Check sheet for the drawn part. Datum: minimum x, y, z corner. Units: mm. Give positions to 0.01 mm unless a question says otherwise; leave off trailing zeros. Order: outer loops, then holes, each group sorted by start corner. A loop starts at its lowest first (then second) coordinate and runs counter-clockwise, first axis right, second up. Notation, with made-up numbers: (-0.75, -12.75) -> (8.25, -12.75) arc R30 ccw to (8.25, 13.25) -> close; hole circle Ø1 at (53.5, 21.5). An arc over 180 degrees is marked (long way). Answer in a Markdown table with one row per item. Add a question column.
(1) Cross-section at B-B (x = 71.5). Record the cut outline in (y, z), then the cut area to 3 significant figures.
(2) Cross-section at C-C (z = 36). Record the cut outline in (x, y), then the cut area to 3 significant figures.
(3) Release check for a two-part mould opening along X. For the marked faces 1 and 2 record: released by +X, released by -X, zero draft, split by the parting line, or undercut.
(4) Cross-section at D-D (z = 46.5). Record the cut outline in (x, y), then the cut area to 3 significant figures.
(5) Go/stop test with flat-tipped pins: pin 1 (2 mm diameter, centred on x = 32.5, y = 1.5, fed in from -Z); pin 2 (5.5 mm diameter, centred on x = 71.5, z = 46.5, fed in from +Y); pin 3 (2 mm diameter, centred on x = 26.5, z = 25.5, fed in from +Y). Record where each tip stops, or that it passes through.
(6) Thickness scan on L1, parallel to X at y = 3.6, z = 46.5; L2, parallel to X at y = 3, z = 38; L3, parallel to Z at x = 21.5, y = 5.5. Record the ranges inside material, lowest first. Write a range as [from, to].
(7) Cross-section at A-A (y = 3). State how many separate pieces and enclosed holes the cut face has, then the cut area to 3 significant figures.
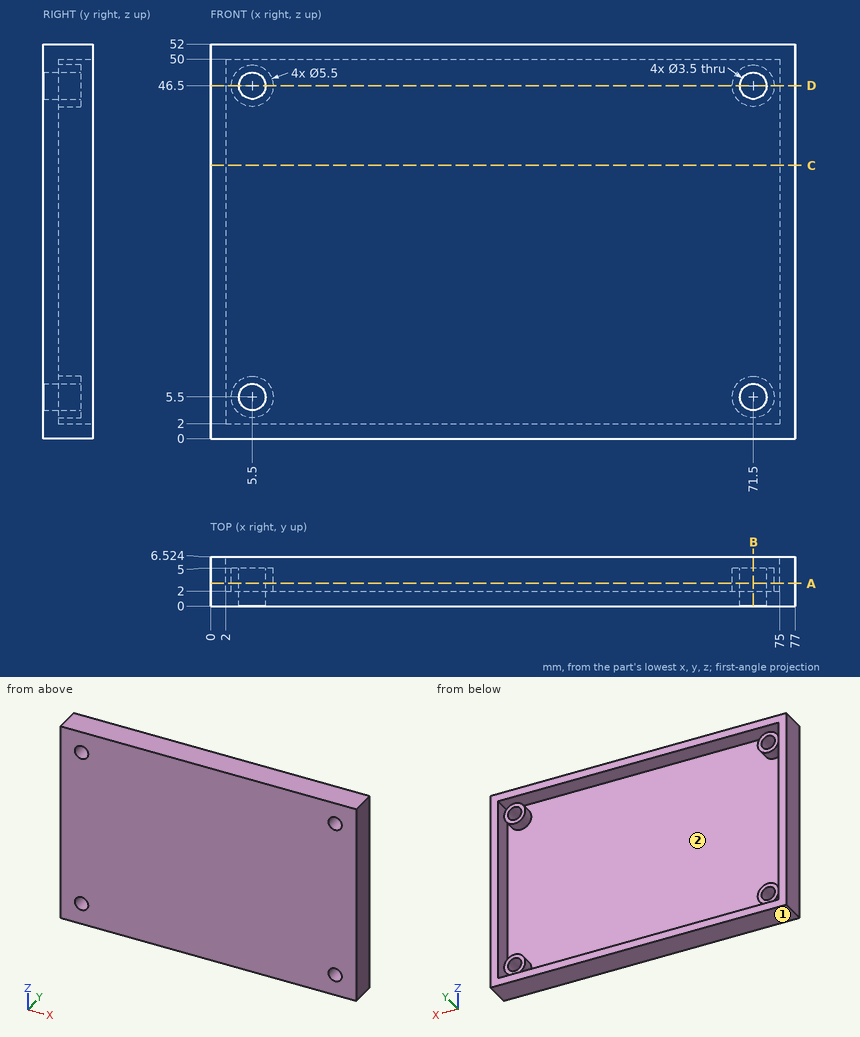
Answer below:
| question | item | result |
|---|---|---|
| 1 | outline | (0, 0) -> (6.52, 0) -> (6.52, 2) -> (2, 2) -> (2, 2.75) -> (5, 2.75) -> (5, 3.75) -> (0, 3.75) -> close; (0, 7.25) -> (5, 7.25) -> (5, 8.25) -> (2, 8.25) -> (2, 43.75) -> (5, 43.75) -> (5, 44.75) -> (0, 44.75) -> close; (0, 48.25) -> (5, 48.25) -> (5, 49.25) -> (2, 49.25) -> (2, 50) -> (6.52, 50) -> (6.52, 52) -> (0, 52) -> close |
| 1 | area | 120 mm² |
| 2 | outline | (0, 0) -> (77, 0) -> (77, 6.52) -> (75, 6.52) -> (75, 2) -> (2, 2) -> (2, 6.52) -> (0, 6.52) -> close |
| 2 | area | 172 mm² |
| 3 | face 1 | zero draft |
| 3 | face 2 | undercut |
| 4 | outline | (0, 0) -> (3.75, 0) -> (3.75, 5) -> (2.75, 5) -> (2.75, 2) -> (2, 2) -> (2, 6.52) -> (0, 6.52) -> close; (7.25, 0) -> (69.75, 0) -> (69.75, 5) -> (68.75, 5) -> (68.75, 2) -> (8.25, 2) -> (8.25, 5) -> (7.25, 5) -> close; (73.25, 0) -> (77, 0) -> (77, 6.52) -> (75, 6.52) -> (75, 2) -> (74.25, 2) -> (74.25, 5) -> (73.25, 5) -> close |
| 4 | area | 170 mm² |
| 5 | pin 1 | stops at z = 0 |
| 5 | pin 2 | stops at y = 5 |
| 5 | pin 3 | stops at y = 2 |
| 6 | L1 | x = [0, 2], [2.75, 3.75], [7.25, 8.25], [68.75, 69.75], [73.25, 74.25], [75, 77] |
| 6 | L2 | x = [0, 2], [75, 77] |
| 6 | L3 | z = [0, 2], [50, 52] |
| 7 | separate pieces | 5 |
| 7 | enclosed holes | 5 |
| 7 | area | 557 mm² |
